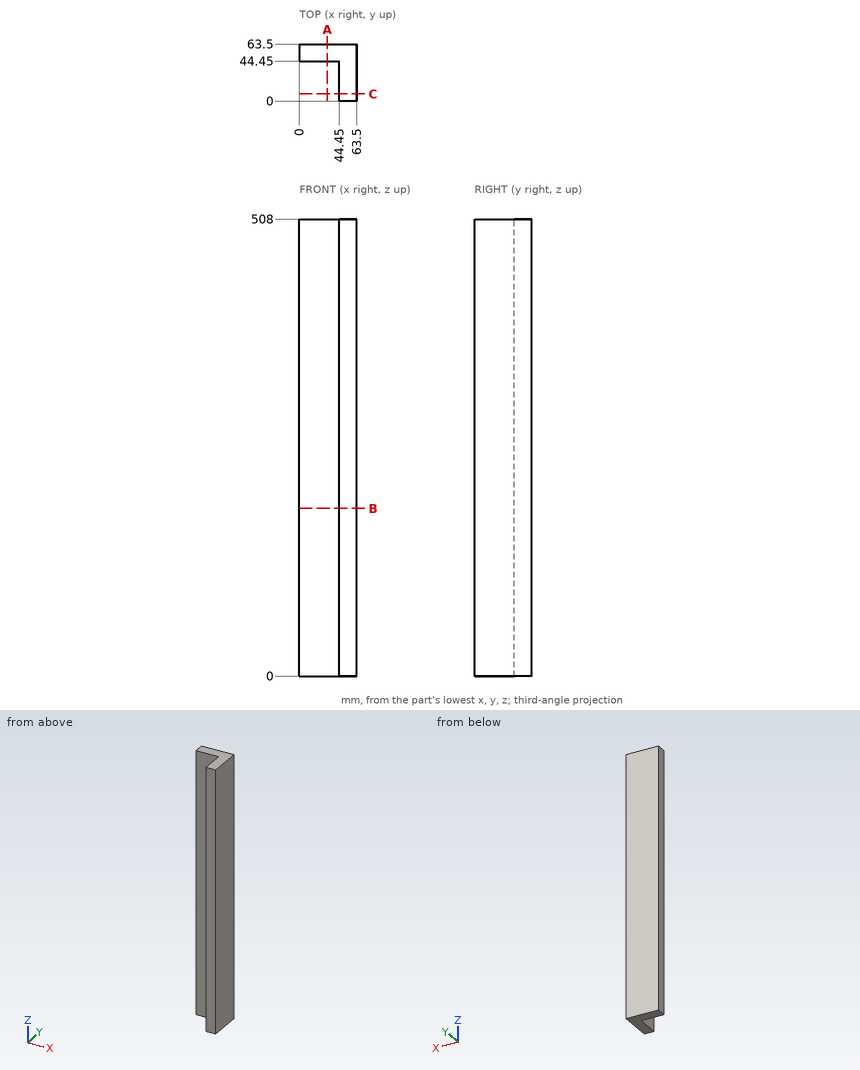
Answer from the drawing. Dimensions are ordinates in mm from the lowest x, y and z of the part. Round coordinates to 2 decimals unless told otherwise and drop trailing zeros. Write each loop counter-clockwise with the first axis right and the second up, starting at its lowest first coordinate (ties: lowest second). Pieces come first, ordered by that corner, then holes. Notation, with made-up numbers: (36.25, 19) - (55.25, 19) arc R9 cw to (55.25, 27) - close; hole circle Ø10 at (31.25, 41.25). An arc over 180 degrees is marked (long way). One line per item, written item: value.
Q1. Find section A-A (x = 31). Determine the outline of the cut face in (y, z).
The answers:
outline: (44.45, 0) - (63.5, 0) - (63.5, 508) - (44.45, 508) - close
Q2. Find section B-B (z = 186.5). Determine the outline of the cut face in (x, y), and give its area (3 significant figures).
The answers:
outline: (0, 44.45) - (44.45, 44.45) - (44.45, 0) - (63.5, 0) - (63.5, 63.5) - (0, 63.5) - close
area: 2,060 mm2
Q3. Each of these flat-tipped pins is pushed along its axis until it touches: P1, Ø22, axis at y = 21, z = 271.5, coming from the -X side; P2, Ø2, axis at x = 29.5, z = 377, coming from the -Y side. Where does it stop, or does it pass through?
The answers:
P1: stops at x = 44.45
P2: stops at y = 44.45
Q4. A straight line is drawn through the part: line 1 (X direction, y = 8.5, z = 147.5). Find the intervals that lie inside material, in ascending order. Write a range as from..to.
The answers:
line 1: x = 44.45..63.5
